Input: part model. Units: mm. Frame: model coordinates. A direction names the side the tool comes from. Coordinates: 2 decimals unless noted, no trailing zeros. Write each loop counter-clockwise with the first axis right and the second up, starting at its lowest first coordinate (ties: lowest second). Pieces come first, ordered by that corner, then holes. Notation, with made-up numbers: (73, 6.5) - (114, 6.5) arc R23 cw to (114, 34.5) - close; hole circle Ø6 at (59, 84.25). An arc over 180 degrees is marked (long way). Use a Markdown table: item, result. Add a question column.
Q1. Mould query, pull axis X, two halves, no side actions, for faces 1 (the face through (-14.09, 1.233, 14.194)), 2 (the face through (21, 0, -22)), 3 (the face through (24.75, 2.5, 14.23)). Classes: released by +X, released by -X, zero draft, split by the parting line, or undercut.
Q2. Section query B-B (y = 3.4). Return the cut outline in (x, z), then the cut area to 3 significant figures.
Q3. Material intervals for probe 1 along Z at (x, y) = (22.5, 1.7); probe 2 along Z at (x, y) = (15.5, 0.45); probe 3 along X at (y, z) = (1.1, -13.5), sorted ascending. Write a range as from..to.
Q4. Set-up query: faces 4 (the face through (5.106, 1.233, -19.337)), 5 (the face through (-28, 0, -8)). Return all of +Z, -Z, +X, -X, +Y, -Y with unobstructed straight access to the full face (end or side cutting, diameter ignored); none if empty.
Q5. Section query A-A (x = -6.5). Return the cut outline in (y, z), then the cut area to 3 significant figures.
Q6. Pin query (flat end, axial travel): P1, Ø4, axis at x = 8, z = 1, coming from the -Y side; P2, Ø1.5, axis at y = 4.5, z = 2.5, coming from the +X side; P3, Ø1.5, axis at x = -27, y = 2, coming from the +Z side. Return the tip coordinate at first contact, or that it passes through.
from build123d import *

# Parameters (mm, degrees)
SKETCH_1_W               = 2.5
SKETCH_1_H               = 60
EXTRUDE_1_DEPTH          = 5
EXTRUDE_2_DEPTH          = 5
CUT_EXTRUDE_START        = -60
SKETCH_4_R               = 2.5
CUT_EXTRUDE_1_DEPTH      = 60
PATTERN_CIRCULAR_2_COUNT = 12
SKETCH_5_R               = 20
CUT_EXTRUDE_2_DEPTH      = 2.5


with BuildPart() as part:
    # Эскиз1 → Повернуть2 (revolve)
    with BuildSketch(Plane(origin=(0, 0, 0), x_dir=(1, 0, 0), z_dir=(0, 1, 0)), mode=Mode.PRIVATE) as revolve_2_sk:
        with Locations((-1.25, 30)):
            Rectangle(SKETCH_1_W, SKETCH_1_H)
    revolve(revolve_2_sk.sketch.rotate(Axis((0, 0, 37.5), (0, 0, -1)), 180), axis=Axis((0, 0, 37.5), (0, 0, -1)))

    # Эскиз1<5> → Бобышка-Вытянуть1 (add)
    with BuildSketch(Plane(origin=(0, 0, 0), x_dir=(1, 0, 0), z_dir=(0, 1, 0))):
        with BuildLine():
            ThreePointArc((20, 0), (-13.228756555, -15), (-2.5, 19.843134833))
            Line((-2.5, 19.843134833), (-2.5, 37.416573868))
            ThreePointArc((-2.5, 37.416573868), (-25.617376915, -27.386127875), (37.5, 0))
            ThreePointArc((37.5, 0), (26.516504294, 26.516504294), (0, 37.5))
            Line((0, 37.5), (0, 20))
            ThreePointArc((0, 20), (14.142135624, 14.142135624), (20, 0))
        make_face()
        with BuildLine():
            Line((-2.5, 37.416573868), (-2.5, 19.843134833))
            ThreePointArc((-2.5, 19.843134833), (-1.252458251, 19.960745185), (0, 20))
            Line((0, 20), (0, 37.5))
            ThreePointArc((0, 37.5), (-1.250695798, 37.479137664), (-2.5, 37.416573868))
        make_face()
    extrude(amount=EXTRUDE_1_DEPTH)

    # Эскиз1<6> → Бобышка-Вытянуть2 (add)
    with BuildSketch(Plane(origin=(0, 0, 0), x_dir=(1, 0, 0), z_dir=(0, 1, 0))):
        with BuildLine():
            Line((0, 0), (-2.5, 0))
            Line((-2.5, 0), (-2.5, 19.843134833))
            ThreePointArc((-2.5, 19.843134833), (-13.228756555, -15), (20, 0))
            ThreePointArc((20, 0), (14.142135624, 14.142135624), (0, 20))
            Line((0, 20), (0, 0))
        make_face()
        with BuildLine():
            Line((-2.5, 19.843134833), (-2.5, 0))
            Line((-2.5, 0), (0, 0))
            Line((0, 0), (0, 20))
            ThreePointArc((0, 20), (-1.252458251, 19.960745185), (-2.5, 19.843134833))
        make_face()
    extrude(amount=EXTRUDE_2_DEPTH)

    # Эскиз4 → Вырез-Вытянуть1 (cut)
    with BuildSketch(Plane(origin=(0, 0, -60), x_dir=(-1, 0, 0), z_dir=(0, 0, -1)).offset(CUT_EXTRUDE_START)):
        Circle(SKETCH_4_R)
    cut_extrude_1 = extrude(amount=CUT_EXTRUDE_1_DEPTH, mode=Mode.SUBTRACT)

    # Круговой массив2: Вырез-Вытянуть1 ×12 about axis
    pattern_circular_2_axis = Axis((0, 29.957095594, 0), (0, -1, 0))
    for i in range(1, PATTERN_CIRCULAR_2_COUNT):
        add(cut_extrude_1.rotate(pattern_circular_2_axis, i * 360 / PATTERN_CIRCULAR_2_COUNT), mode=Mode.SUBTRACT)

    # Эскиз5 → Вырез-Вытянуть2 (cut)
    with BuildSketch(Plane.XZ):
        Circle(SKETCH_5_R)
    extrude(amount=-CUT_EXTRUDE_2_DEPTH, mode=Mode.SUBTRACT)


solid = part.part
Values follow:
| question | item | result |
|---|---|---|
| 1 | face 1 | undercut |
| 1 | face 2 | zero draft |
| 1 | face 3 | undercut |
| 2 | outline | circle Ø75 at (0, 0) |
| 2 | area | 4,420 mm2 |
| 3 | probe 1 | -30..-15.11, -10.87..-1.83, 1.83..10.87, 15.11..30 |
| 3 | probe 2 | -34.15..-31.77, -21.93..-12.64, 12.64..21.93, 31.77..34.15 |
| 3 | probe 3 | -34.99..-27.87, -18.89..-14.76, 14.76..18.89, 27.87..34.99 |
| 4 | face 4 | -Y |
| 4 | face 5 | +Z, -Z, +X, -X, -Y |
| 5 | outline | (0, -36.93) - (5, -36.93) - (5, 36.93) - (0, 36.93) - (0, 18.91) - (2.5, 18.91) - (2.5, -18.91) - (0, -18.91) - close |
| 5 | area | 275 mm2 |
| 6 | P1 | y = 2.5 |
| 6 | P2 | x = 37.46 |
| 6 | P3 | z = 26.78 |
